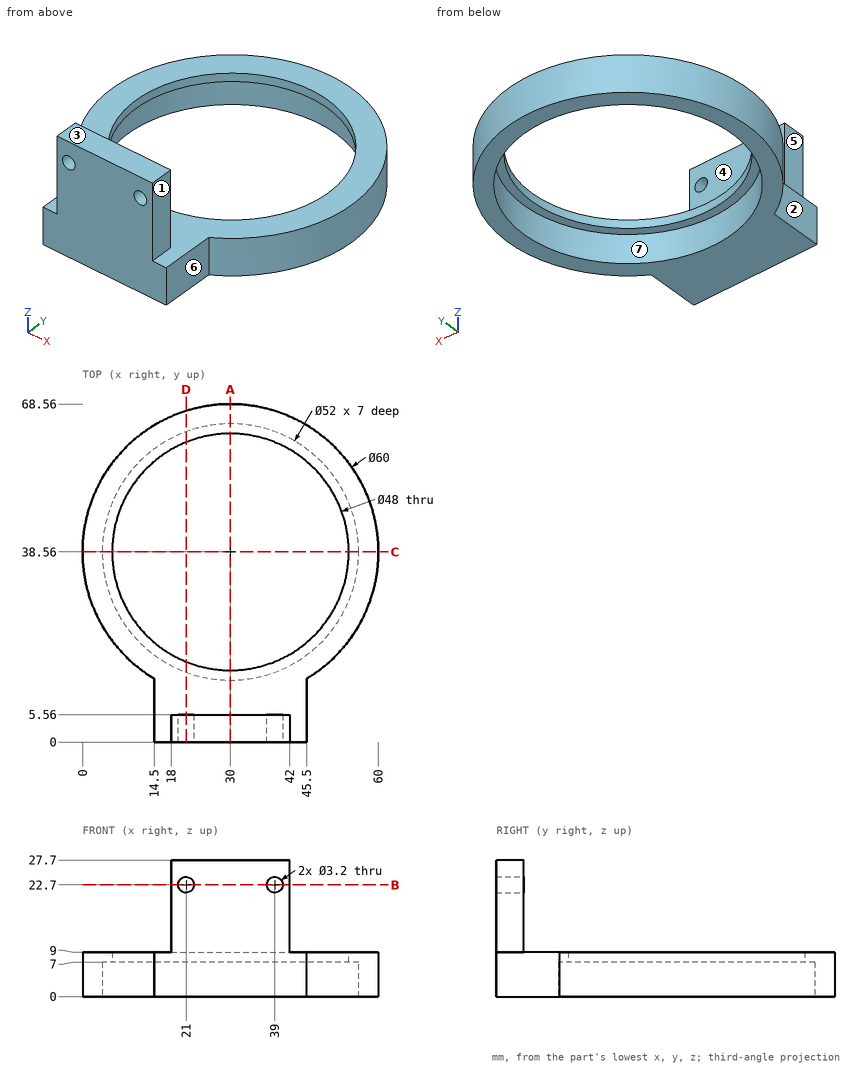
Print and shaded views of the part. All mm, measured from the part's lowest x, y and z. A direction names the side the tool comes from. Coordinates: 2 decimals unless noted, no trailing zeros. Order: outer loops, then holes, each group sorted by start corner. A loop starts at its lowest first (then second) coordinate and runs counter-clockwise, first axis right, second up. Notation, with made-up numbers: M 78.25,-24 L 99.25,-24 A17 ccw 99.25,6 Z; hole C 3.5,-24 d8. An arc over 180 degrees is marked long. Answer as CSV lines item,"result".
1) Cut at B-B (z = 22.7). List the corners of the cut face in (x, y).
Verdict:
outline,"M 18,0 L 19.4,0 L 19.4,5.56 L 18,5.56 Z; M 22.6,0 L 37.4,0 L 37.4,5.56 L 22.6,5.56 Z; M 40.6,0 L 42,0 L 42,5.56 L 40.6,5.56 Z"
2) Flat gauge pins, fed straight in: P1, Ø1.9, axis at x = 39, z = 22.7, coming from the -Y side; P2, Ø3, axis at y = 51, z = 4.5, coming from the +X side; P3, Ø3, axis at y = 2.5, z = 19.5, coming from the -X side; P4, Ø4.5, axis at y = 3, z = 22.5, coming from the +X side. Where does each tip first touch, or does it go through?
Verdict:
P1,"through"
P2,"x = 57.93"
P3,"x = 18"
P4,"x = 42"
3) Drill centre lines: L1, parallel to X at y = 2.9, z = 22.7; L2, parallel to Z at x = 21, y = 2; L3, parallel to Y at x = 30, z = 8.05. Where is each one in solid material? Low to high. Write a range as from..to.
Verdict:
L1,"18..19.4, 22.6..37.4, 40.6..42"
L2,"0..21.1, 24.3..27.7"
L3,"0..14.56, 62.56..68.56"
4) Cut at A-A (x = 30). List the corners of the cut face in (y, z).
Verdict:
outline,"M 0,0 L 12.56,0 L 12.56,7 L 14.56,7 L 14.56,9 L 5.56,9 L 5.56,27.7 L 0,27.7 Z; M 62.56,7 L 64.56,7 L 64.56,0 L 68.56,0 L 68.56,9 L 62.56,9 Z"
5) Mould opens along X. For the marked faces 4, 5, 6 and 7 say: released by +X, released by -X, zero draft, split by the parting line, or undercut.
Verdict:
face 4,"zero draft"
face 5,"released by -X"
face 6,"released by +X"
face 7,"undercut"
6) Cut at D-D (x = 21). List the corners of the cut face in (y, z).
Verdict:
outline,"M 0,0 L 14.17,0 L 14.17,7 L 16.31,7 L 16.31,9 L 5.56,9 L 5.56,21.1 L 0,21.1 Z; M 0,24.3 L 5.56,24.3 L 5.56,27.7 L 0,27.7 Z; M 60.81,7 L 62.95,7 L 62.95,0 L 67.18,0 L 67.18,9 L 60.81,9 Z"
7) 3-axis set-ups, long thin cutter, end or side, ignore diameter. For the marked faces 1, 2 and 3: which of +Z, -Z, +X, -X, +Y, -Y reach the whole face in a straight line?
Verdict:
face 1,"+Z, +X, +Y, -Y"
face 2,"+Z, -Z, -X, -Y"
face 3,"+Z, +X, -X, +Y, -Y"
8) Cut at C-C (y = 38.56). List the corners of the cut face in (x, z), then the cut area to 3 significant figures.
Verdict:
outline,"M 0,0 L 4,0 L 4,7 L 6,7 L 6,9 L 0,9 Z; M 54,7 L 56,7 L 56,0 L 60,0 L 60,9 L 54,9 Z"
area,"80.0 mm2"
